Geometry check sheet. Reference: the model listing, model coordinates, mm. Face numbers are marked on the shaded views. Coordinates: 2 decimals unless noted, no trailing zeros. Loops run counter-clockwise (first coordinate to the right, second up) from the corner with the lowest first, then second, coordinate; pieces in that order, holes last. Notation, with made-up numbers: (-34, 19.25) - (-27, 19.25) arc R9 cw to (-27, 33.25) - close; hole circle Ø2 at (84, 16.5). An arc over 180 degrees is marked (long way). One line per item, written item: value.
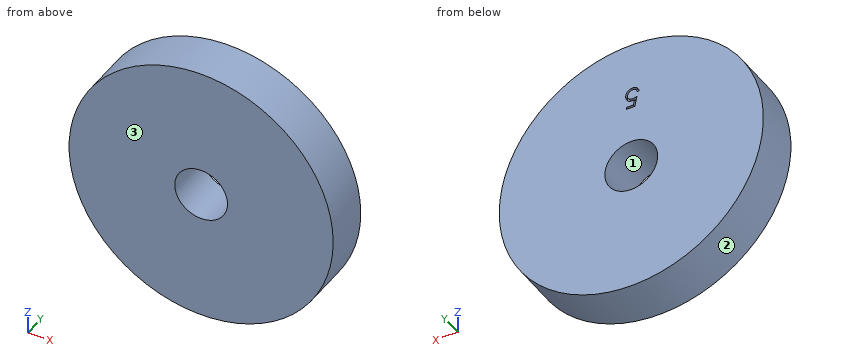
from build123d import *

# Parameters (mm, degrees)
ESQUISSE1_R             = 22.5
BOSS_EXTRU_1_DEPTH      = 8
ESQUISSE2_R             = 4.5
ENL_V_MAT_EXTRU_1_DEPTH = 8
ENL_V_MAT_EXTRU_2_DEPTH = 0.5


with BuildPart() as part:
    # Esquisse1 → Boss.-Extru.1 (new body)
    with BuildSketch(Plane(origin=(0, 0, 0), x_dir=(1, 0, 0), z_dir=(0, 1, 0))):
        Circle(ESQUISSE1_R)
    extrude(amount=BOSS_EXTRU_1_DEPTH)

    # Esquisse2 → Enlèv. mat.-Extru.1 (cut)
    with BuildSketch(Plane(origin=(0, 8, 0), x_dir=(1, 0, 0), z_dir=(0, 1, 0))):
        Circle(ESQUISSE2_R)
    extrude(amount=-ENL_V_MAT_EXTRU_1_DEPTH, mode=Mode.SUBTRACT)

    # Esquisse3 → Enlèv. mat.-Extru.2 (cut)
    with BuildSketch(Plane(origin=(0, 8, 0), x_dir=(1, 0, 0), z_dir=(0, 1, 0))):
        with BuildLine():
            Line((0.827199958, -10.808267064), (0.827199958, -11.167241423))
            Line((0.827199958, -11.167241423), (-0.36330485, -11.167241423))
            Line((-0.36330485, -11.167241423), (-0.551906612, -12.08781434))
            add(Edge.make_bspline(
                [(-0.551906612, -12.08781434), (-0.514850738, -12.077584068), (-0.443060842, -12.057764534), (-0.337100981, -12.035758764), (-0.236508778, -12.02249332), (-0.171233407, -12.020682009), (-0.139646997, -12.019805526)],
                knots=[0, 0, 0, 0, 0.000115302, 0.000223379, 0.000324431, 0.000419176, 0.000419176, 0.000419176, 0.000419176], degree=3))
            add(Edge.make_bspline(
                [(-0.139646997, -12.019805526), (-0.100563257, -12.020651461), (-0.02371486, -12.022314782), (0.088724087, -12.038286632), (0.19605698, -12.063426546), (0.29805935, -12.098547068), (0.394919901, -12.143456801), (0.485747463, -12.199556742), (0.571905376, -12.265090073), (0.65184797, -12.340435085), (0.724372278, -12.423356702), (0.788138267, -12.512514573), (0.842300858, -12.607042235), (0.885861613, -12.707842843), (0.920645947, -12.813801997), (0.943797942, -12.926034579), (0.959214651, -13.043482699), (0.960937037, -13.123787269), (0.961815343, -13.164737417)],
                knots=[0, 0, 0, 0, 0.00011719, 0.000230425, 0.000339944, 0.000447481, 0.000553499, 0.000659556, 0.000767111, 0.000877722, 0.000988528, 0.001097091, 0.001206056, 0.001314692, 0.001425996, 0.001539995, 0.001658004, 0.001780798, 0.001780798, 0.001780798, 0.001780798], degree=3))
            add(Edge.make_bspline(
                [(0.961815343, -13.164737417), (0.961150268, -13.193259637), (0.959829105, -13.249918625), (0.953110517, -13.334062825), (0.940174801, -13.416425658), (0.922807077, -13.49701805), (0.900264659, -13.575687422), (0.872975605, -13.65265895), (0.839579578, -13.727453557), (0.802948202, -13.800778952), (0.761701724, -13.870977459), (0.715923217, -13.936626446), (0.667557726, -13.998710727), (0.61551634, -14.05656446), (0.559315345, -14.109807478), (0.499635378, -14.15875576), (0.436952659, -14.20423709), (0.370297417, -14.244405285), (0.301154934, -14.281368241), (0.228526717, -14.311691779), (0.154066016, -14.338802307), (0.076701141, -14.360411834), (-0.003392672, -14.377344389), (-0.086347447, -14.38884499), (-0.171728117, -14.397221427), (-0.22960313, -14.397745784), (-0.258837702, -14.398010654)],
                knots=[0, 0, 0, 0, 8.5583e-05, 0.000170009, 0.000253005, 0.000335518, 0.000417186, 0.000498352, 0.000580291, 0.000662755, 0.000744161, 0.000824288, 0.000902692, 0.000980133, 0.001057498, 0.001134702, 0.00121156, 0.001289599, 0.001368002, 0.001446531, 0.001525481, 0.001605609, 0.001687289, 0.001770875, 0.001856759, 0.001944425, 0.001944425, 0.001944425, 0.001944425], degree=3))
            add(Edge.make_bspline(
                [(-0.258837702, -14.398010654), (-0.293711883, -14.397319816), (-0.362322713, -14.395960674), (-0.462843281, -14.381742189), (-0.559557886, -14.361378272), (-0.651687987, -14.330742002), (-0.740059251, -14.292354708), (-0.823481969, -14.243838536), (-0.904087745, -14.188859432), (-0.978599782, -14.123979079), (-1.047755895, -14.053063397), (-1.109662404, -13.976105756), (-1.164795981, -13.894376314), (-1.212273728, -13.80747816), (-1.252771749, -13.715639629), (-1.284586737, -13.618516628), (-1.310265092, -13.516616624), (-1.321128513, -13.446463114), (-1.326646196, -13.410831167)],
                knots=[0, 0, 0, 0, 0.000104552, 0.000205693, 0.000304023, 0.000400691, 0.00049644, 0.000592535, 0.000689779, 0.000788716, 0.000888377, 0.000986596, 0.001084603, 0.001183757, 0.001283279, 0.001385267, 0.001490017, 0.001598135, 0.001598135, 0.001598135, 0.001598135], degree=3))
            Line((-1.326646196, -13.410831167), (-1.012543632, -13.410831167))
            add(Edge.make_bspline(
                [(-1.012543632, -13.410831167), (-1.004815074, -13.444207619), (-0.989960358, -13.508359014), (-0.957354609, -13.598490355), (-0.917488734, -13.678809579), (-0.870084385, -13.750379162), (-0.813534355, -13.81278816), (-0.749004926, -13.868405221), (-0.676657202, -13.918580351), (-0.596263973, -13.960403118), (-0.511450894, -13.996071871), (-0.422683684, -14.019823566), (-0.332379337, -14.036524459), (-0.271300967, -14.03819622), (-0.240608535, -14.039036295)],
                knots=[0, 0, 0, 0, 0.000102709, 0.000197412, 0.000286774, 0.000371169, 0.000454082, 0.000538572, 0.000626283, 0.000717552, 0.000809994, 0.00090168, 0.00099274, 0.001084718, 0.001084718, 0.001084718, 0.001084718], degree=3))
            add(Edge.make_bspline(
                [(-0.240608535, -14.039036295), (-0.210650091, -14.038215517), (-0.151661669, -14.036599399), (-0.064850282, -14.024160386), (0.018962592, -14.005002815), (0.098949949, -13.97633296), (0.176511488, -13.941488242), (0.249685259, -13.896773166), (0.320588136, -13.845313148), (0.38701627, -13.786356517), (0.447855719, -13.721386823), (0.50161184, -13.651909429), (0.546388753, -13.577792583), (0.584122862, -13.50031943), (0.612776161, -13.418640873), (0.633217142, -13.333139698), (0.645220201, -13.243604717), (0.646871381, -13.182535408), (0.647712779, -13.151416103)],
                knots=[0, 0, 0, 0, 8.9842e-05, 0.0001769, 0.000262612, 0.000347317, 0.000431396, 0.000517249, 0.000604055, 0.000693954, 0.000783242, 0.000870748, 0.000956963, 0.001042571, 0.001128832, 0.00121607, 0.001305907, 0.001399251, 0.001399251, 0.001399251, 0.001399251], degree=3))
            add(Edge.make_bspline(
                [(0.647712779, -13.151416103), (0.647054299, -13.123340351), (0.645765419, -13.068386062), (0.635234849, -12.987986855), (0.616917877, -12.911913813), (0.591493997, -12.839799579), (0.559214489, -12.771576137), (0.519768177, -12.707173077), (0.472414779, -12.647439243), (0.41832289, -12.59234669), (0.359064849, -12.541501815), (0.293621107, -12.498157728), (0.22336118, -12.461693811), (0.14913158, -12.430225812), (0.069166682, -12.407625067), (-0.014949951, -12.390657182), (-0.104126659, -12.380841819), (-0.165097347, -12.379479931), (-0.196437862, -12.378779885)],
                knots=[0, 0, 0, 0, 8.4208e-05, 0.000164824, 0.000242709, 0.000318547, 0.000393815, 0.000468731, 0.000544614, 0.00062196, 0.000700062, 0.000778428, 0.000856831, 0.000937299, 0.001019835, 0.001105635, 0.00119452, 0.001288536, 0.001288536, 0.001288536, 0.001288536], degree=3))
            add(Edge.make_bspline(
                [(-0.196437862, -12.378779885), (-0.223566791, -12.379360476), (-0.279581146, -12.380559249), (-0.365503973, -12.389385746), (-0.455795696, -12.40362504), (-0.550110192, -12.423211288), (-0.6487307, -12.448842365), (-0.751449101, -12.479556865), (-0.858481367, -12.516278864), (-0.930599092, -12.544011078), (-0.967671837, -12.558267064)],
                knots=[0, 0, 0, 0, 8.1378e-05, 0.000168026, 0.000258858, 0.000355524, 0.000456875, 0.000564457, 0.000677092, 0.000796243, 0.000796243, 0.000796243, 0.000796243], degree=3))
            Line((-0.967671837, -12.558267064), (-0.608697478, -10.808267064))
            Line((-0.608697478, -10.808267064), (0.827199958, -10.808267064))
        make_face()
    extrude(amount=-ENL_V_MAT_EXTRU_2_DEPTH, mode=Mode.SUBTRACT)


solid = part.part
(1) Material ranges on probe 1 along Z at (x, y) = (0, 3); probe 2 along Z at (x, y) = (-4, 1.5), recorded low to high. Write a range as from..to.
Reply:
probe 1: -22.5..-4.5, 4.5..22.5
probe 2: -22.14..-2.06, 2.06..22.14
(2) Cross-section at D-D on z = 17.5. Record the cut outline in (x, y), and give its area (3 significant figures).
Reply:
outline: (-14.14, 0) - (14.14, 0) - (14.14, 8) - (-14.14, 8) - close
area: 226 mm2
(3) Cross-section at C-C on y = 4. Record the cut outline in (x, z).
Reply:
outline: circle Ø45 at (0, 0); hole circle Ø9 at (0, 0)
(4) Cross-section at B-B on x = -3. Record the cut outline in (y, z).
Reply:
outline: (0, -22.3) - (8, -22.3) - (8, -3.35) - (0, -3.35) - close; (0, 3.35) - (8, 3.35) - (8, 22.3) - (0, 22.3) - close
(5) Go/stop test with flat-tipped pins: pin 1 Ø12 at (x, z) = (-11.5, -12.5) entering from -Y; pin 2 Ø4 at (y, z) = (1, -10) entering from -X; pin 3 Ø4 at (x, y) = (-16.5, 1) entering from +Z; pin 4 Ø4 at (x, y) = (3, 3) entering from -Z. Record where each tip stops, or that it passes through.
Reply:
pin 1: y = 0
pin 2: x = -21.03
pin 3: z = 17.2
pin 4: z = -22.48
(6) Cross-section at A-A on z = 0. Record the cut outline in (x, y), and give its area (3 significant figures).
Reply:
outline: (-22.5, 0) - (-4.5, 0) - (-4.5, 8) - (-22.5, 8) - close; (4.5, 0) - (22.5, 0) - (22.5, 8) - (4.5, 8) - close
area: 288 mm2
(7) Release check for a two-part mould opening along Z. For the marked faces 1, 2 and 3 record: pulls with the +Z half, pulls with the -Z half, needs draft (parallel to the pull), parting line crosses it, or undercut.
Reply:
face 1: undercut
face 2: parting line crosses it
face 3: needs draft
